For this review, take the finished solid that the model builds, in its own axes (mm). Face numbers are marked on the shaded views. A direction names the side the tool comes from. Give positions to 0.01 mm unless a question says otherwise; leave off trailing zeros. Loops run counter-clockwise (first coordinate to the right, second up) from the corner with the lowest first, then second, coordinate; pieces in that order, holes last.
```python
from build123d import *

# Parameters (mm, degrees)
SKETCH4_W           = 290
SKETCH4_H           = 145
BOSS_EXTRUDE3_DEPTH = 111
SKETCH5_W           = 286
SKETCH5_H           = 141
CUT_EXTRUDE2_DEPTH  = 110.8


with BuildPart() as part:
    # Sketch4 → Boss-Extrude3 (new body)
    with BuildSketch(Plane(origin=(0, 0, 0), x_dir=(1, 0, 0), z_dir=(0, 1, 0))):
        Rectangle(SKETCH4_W, SKETCH4_H)
    extrude(amount=BOSS_EXTRUDE3_DEPTH)

    # Sketch5 → Cut-Extrude2 (cut)
    with BuildSketch(Plane(origin=(0, 0, 0), x_dir=(1, 0, 0), z_dir=(0, 1, 0))):
        Rectangle(SKETCH5_W, SKETCH5_H)
    extrude(amount=CUT_EXTRUDE2_DEPTH, mode=Mode.SUBTRACT)


solid = part.part
```
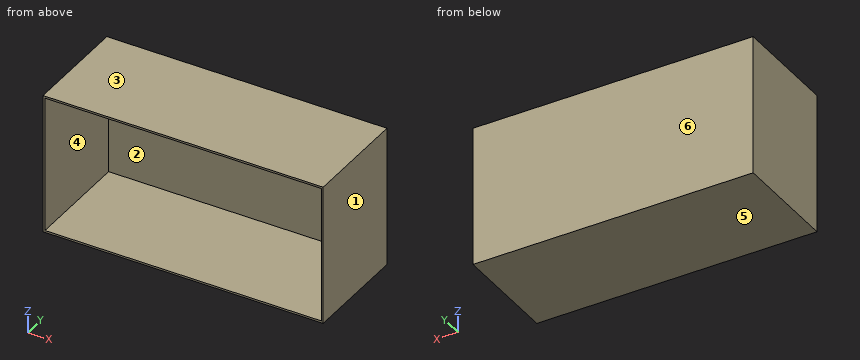
Item 1: Clearance check with a flat-ended pin moving along its axis: pin 1 Ø1 at (x, z) = (-61.5, -41) entering from -Y. State where the tip first meets the part, or that it passes through.
Answer:
pin 1: stops at y = 110.8
Item 2: Take a section at A-A on y = 34. Give the boundary of the cut face in (x, z), and give its area (3 significant figures).
Answer:
outline: (-145, -72.5) - (145, -72.5) - (145, 72.5) - (-145, 72.5) - close; hole (-143, -70.5) - (143, -70.5) - (143, 70.5) - (-143, 70.5) - close
area: 1,720 mm2
Item 3: The part is to be moulded in two halves that separate along Z. For the marked faces 3, 4, 5 and 6, say which applies: released by +Z, released by -Z, zero draft, split by the parting line, or undercut.
Answer:
face 3: released by +Z
face 4: undercut
face 5: released by -Z
face 6: zero draft
Item 4: For L1, parallel to Z at x = 86, y = 63; L2, parallel to X at y = 30.5, z = -6.5; L3, parallel to Y at x = 120, z = 36.5, list the stretches that pass through material, from the lowest coordinate up.
Answer:
L1: z = -72.5 to -70.5, 70.5 to 72.5
L2: x = -145 to -143, 143 to 145
L3: y = 110.8 to 111
Item 5: Take a section at B-B on z = -7. Give the boundary of the cut face in (x, y), and give its area (3 significant figures).
Answer:
outline: (-145, 0) - (-143, 0) - (-143, 110.8) - (143, 110.8) - (143, 0) - (145, 0) - (145, 111) - (-145, 111) - close
area: 501 mm2
Item 6: Take a section at C-C on x = 54. Give the boundary of the cut face in (y, z).
Answer:
outline: (0, -72.5) - (111, -72.5) - (111, 72.5) - (0, 72.5) - (0, 70.5) - (110.8, 70.5) - (110.8, -70.5) - (0, -70.5) - close
Item 7: Tool access review of the marked faces 1 and 2: name each direction out of +Z, -Z, +X, -X, +Y, -Y from which nothing blocks a thin tool from reaching the whole face with its end or side.
Answer:
face 1: +Z, -Z, +X, +Y, -Y
face 2: -Y
